from build123d import *

# Parameters (mm, degrees)
EXTRUDE_1_DEPTH     = 8
SKETCH_2_R          = 1.5
CUT_EXTRUDE_1_DEPTH = 23.912878475
SKETCH_3_R          = 1.5
CUT_EXTRUDE_2_DEPTH = 24.34523506


with BuildPart() as part:
    # 草图1 → 凸台-拉伸1 (new body)
    with BuildSketch(Plane(origin=(0, 0, 0), x_dir=(0, 0, -1), z_dir=(1, 0, 0))):
        Polygon((0, 0), (10, 0), (10, 1), (1, 1), (1, 20), (0, 20), align=None)
    extrude(amount=EXTRUDE_1_DEPTH)

    # 草图2 → 切除-拉伸1 (cut, through all)
    with BuildSketch(Plane(origin=(0, 1, 0), x_dir=(1, 0, 0), z_dir=(0, 1, 0))):
        with Locations(Location((4, 6, 0), (0, 0, 270))):
            Circle(SKETCH_2_R)
    extrude(amount=-CUT_EXTRUDE_1_DEPTH, mode=Mode.SUBTRACT)

    # 草图3 → 切除-拉伸2 (cut, through all)
    with BuildSketch(Plane(origin=(0, 0, -1), x_dir=(-1, 0, 0), z_dir=(0, 0, -1))):
        with Locations(Location((-4, 16, 0), (0, 0, 90))):
            Circle(SKETCH_3_R)
        with Locations(Location((-4, 6, 0), (0, 0, 90))):
            Circle(SKETCH_3_R)
    extrude(amount=-CUT_EXTRUDE_2_DEPTH, mode=Mode.SUBTRACT)


solid = part.part
Could you check a few things on this model? Use its own coordinates, in mm. A direction names the side the tool comes from. Give positions to 0.01 mm unless a question says otherwise; leave off trailing zeros. Order: outer loops, then holes, each group sorted by start corner. A loop starts at its lowest first (then second) coordinate and runs counter-clockwise, first axis right, second up.
Item 1: If we section it at A-A, the plane z = -6: Write out the boundary of the cut face in (x, y), plus the area to 3 significant figures.
Item 2: I need wall thicknesses on line 1 (X direction, y = 6, z = -0.2); line 2 (Z direction, x = 0.5, y = 5); line 3 (Y direction, x = 1.5, z = -2). Which ranges of each line are inside material? Lowest first, please.
Item 3: For faces 5 (the face through (4, 10, -1)), 6 (the face through (4, 0, -4)), which set-ups out of +Z, -Z, +X, -X, +Y, -Y let a thin tool reach every point of the face, with its end or its side?
Item 4: If we section it at D-D, the plane x = 2: Write out the boundary of the cut face in (y, z).
Item 5: If we section it at C-C, the plane y = 16: Write out the boundary of the cut face in (x, z).
Item 6: If we mould it in two halves opening along X, with no side actions, what happens to faces 1 (the face through (8, 7.8, -0.5)), 2 (the face through (4.07, 14.5, -0.51)), 3 (the face through (3.9, 0.5, -10)), 4 (the face through (5.01, 4.89, -0.51))? For each: pulls with the +X half, pulls with the -X half, needs draft (parallel to the pull), parting line crosses it, or undercut.
Item 7: If we section it at B-B, the plane x = 4: Write out the boundary of the cut face in (y, z).
Item 8: I'm going to push flat-ended pins straight in: pin 1 (4 mm diameter, centred on x = 4.5, z = -8.5, fed in from +Y); pin 2 (1.5 mm diameter, centred on x = 3.5, y = 6, fed in from -Z). Where does each tip first touch, or does it pass through?
Values:
1. outline: (0, 0) - (2.5, 0) - (2.5, 1) - (0, 1) - close; (5.5, 0) - (8, 0) - (8, 1) - (5.5, 1) - close
1. area: 5.00 mm2
2. line 1: x = 0 to 2.5, 5.5 to 8
2. line 2: z = -1 to 0
2. line 3: y = 0 to 1
3. face 5: -Z, +X, -X, +Y
3. face 6: +Z, -Z, +X, -X, -Y
4. outline: (0, -10) - (1, -10) - (1, -1) - (20, -1) - (20, 0) - (0, 0) - close
5. outline: (0, -1) - (2.5, -1) - (2.5, 0) - (0, 0) - close; (5.5, -1) - (8, -1) - (8, 0) - (5.5, 0) - close
6. face 1: pulls with the +X half
6. face 2: undercut
6. face 3: needs draft
6. face 4: undercut
7. outline: (0, -10) - (1, -10) - (1, -7.5) - (0, -7.5) - close; (0, -4.5) - (1, -4.5) - (1, -1) - (4.5, -1) - (4.5, 0) - (0, 0) - close; (7.5, -1) - (14.5, -1) - (14.5, 0) - (7.5, 0) - close; (17.5, -1) - (20, -1) - (20, 0) - (17.5, 0) - close
8. pin 1: stops at y = 1
8. pin 2: passes through
